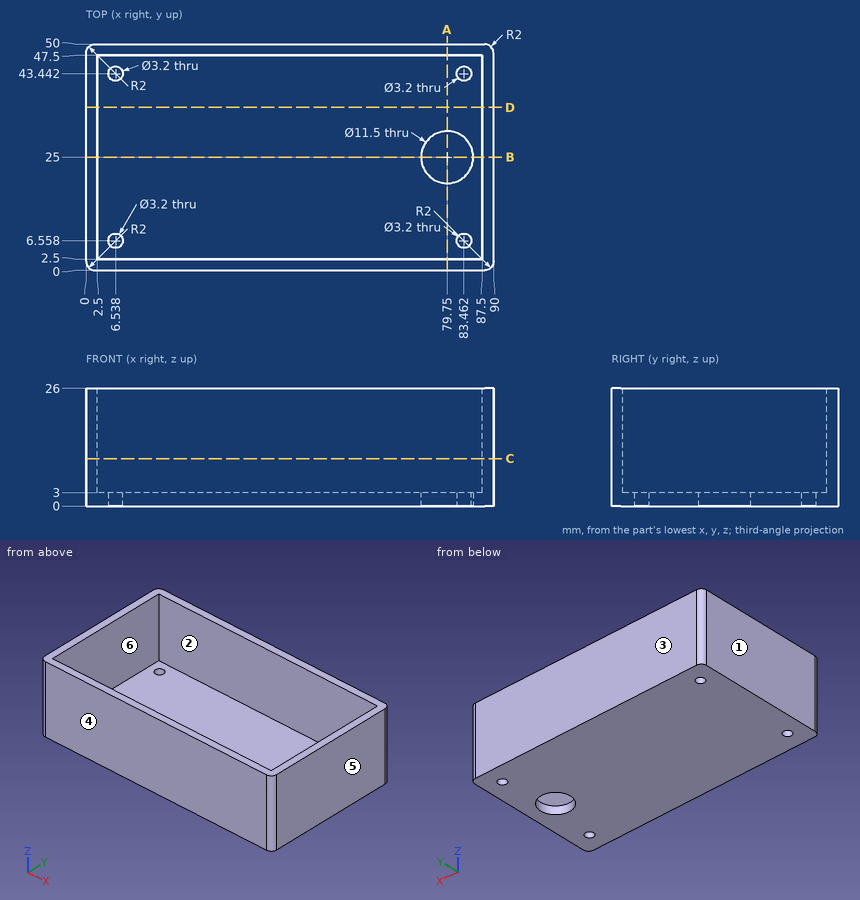
Can you work these out from the drawing? Everything is in mm from the part's minimum corner. A direction names the side the tool comes from. Coordinates: 2 decimals unless noted, no trailing zeros. Loops run counter-clockwise (first coordinate to the right, second up) from the corner with the lowest first, then second, coordinate; pieces in that order, holes last. Notation, with made-up numbers: (-15.75, 47.25) -> (41.25, 47.25) arc R19 ccw to (41.25, 74.25) -> close; hole circle Ø2 at (61.5, 0.25). An arc over 180 degrees is marked (long way). Return JSON: item names as keys, results as strings.
1) For the marked faces 1 and 2, which set-ups out of +Z, -Z, +X, -X, +Y, -Y let a thin tool reach every point of the face, with its end or its side?
Results below:
{"face 1": "+Z, -Z, -X, +Y, -Y", "face 2": "+Z"}
2) Will this pin go through, and if not, where does the flat tip stop? pin 1 (4 mm diameter, centred on x = 83.462, y = 6.558, fed in from +Z).
Results below:
{"pin 1": "z = 3"}
3) If we section it at D-D, the plane y = 36: Write out the boundary of the cut face in (x, z), then the cut area to 3 significant figures.
Results below:
{"outline": "(0, 0) -> (90, 0) -> (90, 26) -> (87.5, 26) -> (87.5, 3) -> (2.5, 3) -> (2.5, 26) -> (0, 26) -> close", "area": "385 mm²"}
4) If we section it at C-C, the plane z = 10.5: Write out the boundary of the cut face in (x, y).
Results below:
{"outline": "(0, 2) arc R2 ccw to (2, 0) -> (88, 0) arc R2 ccw to (90, 2) -> (90, 48) arc R2 ccw to (88, 50) -> (2, 50) arc R2 ccw to (0, 48) -> close; hole (2.5, 2.5) -> (87.5, 2.5) -> (87.5, 47.5) -> (2.5, 47.5) -> close"}
5) Thinking about a two-plate mould opening in Y: for the marked faces 3, 4, 5 and 6, which applies, +Y half, -Y half, draft (parallel to the pull), parting line (faces both ways), or undercut?
Results below:
{"face 3": "+Y half", "face 4": "-Y half", "face 5": "draft", "face 6": "undercut"}
6) If we section it at B-B, the plane y = 25: Write out the boundary of the cut face in (x, z), then the cut area to 4 significant figures.
Results below:
{"outline": "(0, 0) -> (74, 0) -> (74, 3) -> (2.5, 3) -> (2.5, 26) -> (0, 26) -> close; (85.5, 0) -> (90, 0) -> (90, 26) -> (87.5, 26) -> (87.5, 3) -> (85.5, 3) -> close", "area": "350.5 mm²"}
7) If we section it at A-A, the plane x = 79.75: Write out the boundary of the cut face in (y, z).
Results below:
{"outline": "(0, 0) -> (19.25, 0) -> (19.25, 3) -> (2.5, 3) -> (2.5, 26) -> (0, 26) -> close; (30.75, 0) -> (50, 0) -> (50, 26) -> (47.5, 26) -> (47.5, 3) -> (30.75, 3) -> close"}
8) I need wall thicknesses on line 1 (X direction, y = 8.5, z = 22); line 2 (Y direction, x = 53.5, z = 15.5); line 3 (Z direction, x = 61, y = 19). Which ranges of each line are inside material? Lowest first, please. Write a range as from..to.
Results below:
{"line 1": "0..2.5, 87.5..90", "line 2": "0..2.5, 47.5..50", "line 3": "0..3"}
